Part print with two shaded views. Sizes in mm from the minimum x, y, z corner. A direction names the side the tool comes from. Round coordinates to 2 decimals unless told otherwise and drop trailing zeros. Order: outer loops, then holes, each group sorted by start corner. A loop starts at its lowest first (then second) coordinate and runs counter-clockwise, first axis right, second up. Notation, with made-up numbers: M 0,84.25 L 32,84.25 A19 cw 32,109.25 Z; hole C -5.5,50.25 d4. An arc over 180 degrees is marked long. Put each result on its own line as item: value.
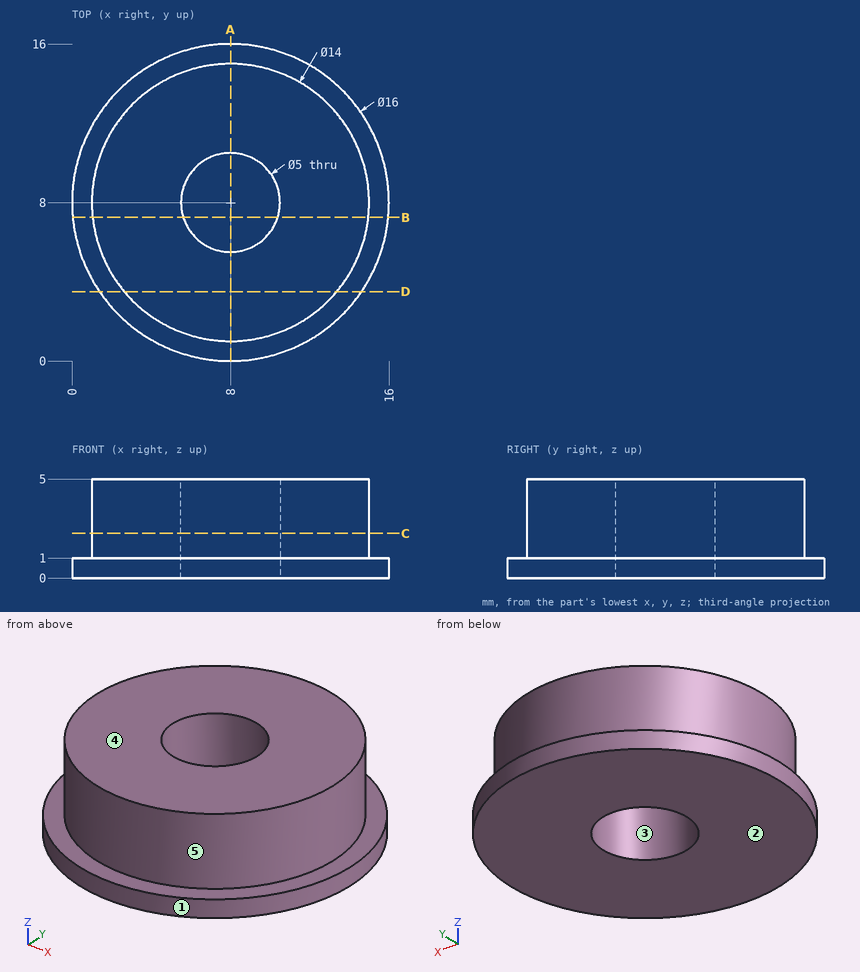
Item 1: Band-saw the part on B-B on y = 7.25. Give the cut face in (x, z), and give its area (3 significant figures).
Answers below:
outline: M 0.04,0 L 5.62,0 L 5.62,5 L 1.04,5 L 1.04,1 L 0.04,1 Z; M 10.38,0 L 15.96,0 L 15.96,1 L 14.96,1 L 14.96,5 L 10.38,5 Z
area: 47.8 mm²
Item 2: Band-saw the part on D-D on y = 3.5. Give the cut face in (x, z).
Answers below:
outline: M 1.39,0 L 14.61,0 L 14.61,1 L 13.36,1 L 13.36,5 L 2.64,5 L 2.64,1 L 1.39,1 Z
Item 3: Probe line 1 along Y through (x, z) = (8, 1.9); line 2 along Z through (x, y) = (14.5, 11.5); line 3 along Y through (x, z) = (9, 1.45). List the from-to ranges inside material, lowest first. Write a range as [from, to].
Answers below:
line 1: [1, 5.5], [10.5, 15]
line 2: [0, 1]
line 3: [1.07, 5.71], [10.29, 14.93]
Item 4: Pin check, flat tips, straight feed: P1, Ø1.5, axis at x = 13, z = 3.5, coming from the +Y side; P2, Ø6.5, axis at x = 8, y = 8, coming from the +Z side. Stop position of each tip, or through.
Answers below:
P1: y = 13.56
P2: z = 5
Item 5: Band-saw the part on C-C on z = 2.25. Give the cut face in (x, y).
Answers below:
outline: C 8,8 d14; hole C 8,8 d5
Item 6: Tool access for the marked faces 4 and 5: list every direction of +Z, -Z, +X, -X, +Y, -Y with a clear straight run to the whole face (end or side of a thin tool).
Answers below:
face 4: +Z, +X, -X, +Y, -Y
face 5: +Z
Item 7: Mould opens along X. For the marked faces 1, 2 and 3 say: pulls with the +X half, pulls with the -X half, needs draft (parallel to the pull), parting line crosses it, or undercut.
Answers below:
face 1: parting line crosses it
face 2: needs draft
face 3: undercut
Item 8: Band-saw the part on A-A on x = 8. Give the cut face in (y, z), and give its area (3 significant figures).
Answers below:
outline: M 0,0 L 5.5,0 L 5.5,5 L 1,5 L 1,1 L 0,1 Z; M 10.5,0 L 16,0 L 16,1 L 15,1 L 15,5 L 10.5,5 Z
area: 47.0 mm²
